```python
from build123d import *

# Parameters (mm, degrees)
BOSS_EXTRUDE1_DEPTH = 5
CUT_EXTRUDE1_DEPTH  = 15
CUT_EXTRUDE4_DEPTH  = 15
SKETCH7_R           = 1
BOSS_EXTRUDE2_DEPTH = 60
SKETCH8_R           = 0.873363885
CUT_EXTRUDE5_DEPTH  = 15
SKETCH9_R           = 0.918957051
CUT_EXTRUDE6_DEPTH  = 15
SKETCH10_R          = 0.859226697
CUT_EXTRUDE7_DEPTH  = 15
SKETCH11_R          = 0.786945752
CUT_EXTRUDE8_DEPTH  = 15


with BuildPart() as part:
    # Sketch1 → Boss-Extrude1 (new body)
    with BuildSketch(Plane(origin=(0, 0, 0), x_dir=(1, 0, 0), z_dir=(0, 1, 0))):
        with BuildLine():
            Line((-35.448928743, 52.732943935), (-27.948927155, 60.232942347))
            ThreePointArc((-27.948927155, 60.232942347), (-7.948927155, 52.732942347), (12.051072845, 60.232942347))
            Line((12.051072845, 60.232942347), (19.551072845, 52.732939171))
            ThreePointArc((19.551072845, 52.732939171), (12.051076647, 32.732945116), (19.551072845, 12.73295106))
            Line((19.551072845, 12.73295106), (12.051060957, 5.232942347))
            ThreePointArc((12.051060957, 5.232942347), (5.043506988, 9.818456658), (-2.948938922, 12.319169055))
            ThreePointArc((-2.948938922, 12.319169055), (-7.948938922, 12.848178709), (-12.948938922, 12.319169055))
            ThreePointArc((-12.948938922, 12.319169055), (-20.941384832, 9.818456658), (-27.9489388, 5.232942347))
            Line((-27.9489388, 5.232942347), (-35.448937212, 12.732943935))
            ThreePointArc((-35.448937212, 12.732943935), (-27.948932978, 32.732942347), (-35.448928743, 52.732943935))
        make_face()
    extrude(amount=BOSS_EXTRUDE1_DEPTH)

    # Sketch3 → Cut-Extrude1 (cut)
    with BuildSketch(Plane(origin=(0, 5, 0), x_dir=(1, 0, 0), z_dir=(0, 1, 0))):
        with BuildLine():
            Line((-27.948927155, 60.232942347), (-35.448928743, 52.732943935))
            ThreePointArc((-35.448928743, 52.732943935), (-27.948932978, 32.732942347), (-35.448937212, 12.732943935))
            Line((-35.448937212, 12.732943935), (-27.9489388, 5.232942347))
            ThreePointArc((-27.9489388, 5.232942347), (-7.948938922, 12.848178709), (12.051060957, 5.232942347))
            Line((12.051060957, 5.232942347), (19.551072845, 12.73295106))
            ThreePointArc((19.551072845, 12.73295106), (12.051076647, 32.732945116), (19.551072845, 52.732939171))
            Line((19.551072845, 52.732939171), (12.051072845, 60.232942347))
            ThreePointArc((12.051072845, 60.232942347), (-7.948927155, 52.732942347), (-27.948927155, 60.232942347))
        make_face()
        with BuildLine():
            Line((-33.493710626, 12.732943935), (-27.9489388, 7.18817211))
            ThreePointArc((-27.9489388, 7.18817211), (-7.948938922, 14.210022681), (12.051060957, 7.18817211))
            Line((12.051060957, 7.18817211), (17.099712422, 12.236821437))
            ThreePointArc((17.099712422, 12.236821437), (10.006359282, 32.484880304), (17.099712422, 52.732939171))
            Line((17.099712422, 52.732939171), (12.051072845, 57.781578748))
            ThreePointArc((12.051072845, 57.781578748), (-7.948927155, 51.108457819), (-27.948927155, 57.781578748))
            Line((-27.948927155, 57.781578748), (-33.493710626, 52.732943935))
            ThreePointArc((-33.493710626, 52.732943935), (-26.205843846, 32.732943935), (-33.493710626, 12.732943935))
        make_face(mode=Mode.SUBTRACT)
    extrude(amount=-CUT_EXTRUDE1_DEPTH, mode=Mode.SUBTRACT)


with BuildPart() as cut_extrude1_kept_piece:
    # of the separate pieces the step leaves, the one the design keeps (cut_extrude1_pieces_kept)
    add(part.part.solids().sort_by_distance((-27.9489388, 0, -7.18817211))[0])

    # Sketch4 → Cut-Extrude4 (cut)
    with BuildSketch(Plane(origin=(0, 5, 0), x_dir=(1, 0, 0), z_dir=(0, 1, 0))):
        with BuildLine():
            Line((-19.583778872, 20.459711597), (-16.194704715, 20.459711597))
            ThreePointArc((-16.194704715, 20.459711597), (-14.85807522, 21.796341092), (-16.194704715, 23.132970587))
            Line((-16.194704715, 23.132970587), (-19.583778872, 23.132970587))
            ThreePointArc((-19.583778872, 23.132970587), (-20.920408367, 21.796341092), (-19.583778872, 20.459711597))
        make_face()
        with BuildLine():
            ThreePointArc((-21.831761669, 21.796341092), (-21.78134565, 17.350791516), (-17.335796074, 17.401207535))
            ThreePointArc((-17.335796074, 17.401207535), (-15.079204869, 17.426799049), (-15.053613355, 15.170207843))
            ThreePointArc((-15.053613355, 15.170207843), (-24.012345341, 15.068608797), (-24.113944388, 24.027340783))
            ThreePointArc((-24.113944388, 24.027340783), (-21.857353183, 24.052932297), (-21.831761669, 21.796341092))
        make_face()
        with BuildLine():
            ThreePointArc((-17.153953535, 47.057082623), (-21.758601657, 47.312085175), (-22.013604209, 42.707437053))
            ThreePointArc((-22.013604209, 42.707437053), (-22.114274365, 40.88960957), (-23.932101848, 40.990279726))
            ThreePointArc((-23.932101848, 40.990279726), (-23.475758984, 49.230582815), (-15.235455895, 48.77423995))
            ThreePointArc((-15.235455895, 48.77423995), (-15.336126051, 46.956412467), (-17.153953535, 47.057082623))
        make_face()
        with BuildLine():
            ThreePointArc((-18.867938752, 44.161713483), (-20.322215182, 42.707437053), (-18.867938752, 41.253160623))
            Line((-18.867938752, 41.253160623), (-17.153953535, 41.253160623))
            ThreePointArc((-17.153953535, 41.253160623), (-15.699677105, 42.707437053), (-17.153953535, 44.161713483))
            Line((-17.153953535, 44.161713483), (-18.867938752, 44.161713483))
        make_face()
        with BuildLine():
            Line((-8.881617516, 44.161713483), (-8.881617516, 19.598774313))
            ThreePointArc((-8.881617516, 19.598774313), (-7.948927155, 18.666083952), (-7.016236793, 19.598774313))
            Line((-7.016236793, 19.598774313), (-7.016236793, 44.161713483))
            ThreePointArc((-7.016236793, 44.161713483), (-7.948927155, 45.094403844), (-8.881617516, 44.161713483))
        make_face()
        with BuildLine():
            Line((-22.013604209, 33.925546285), (5.888104042, 33.925546285))
            ThreePointArc((5.888104042, 33.925546285), (7.080706392, 32.732943935), (5.888104042, 31.540341586))
            Line((5.888104042, 31.540341586), (-22.013604209, 31.540341586))
            ThreePointArc((-22.013604209, 31.540341586), (-23.206206558, 32.732943935), (-22.013604209, 33.925546285))
        make_face()
        with BuildLine():
            ThreePointArc((6.501599793, 42.67386899), (5.971735558, 47.620514921), (1.025089628, 47.090650686))
            ThreePointArc((1.025089628, 47.090650686), (-0.822878242, 46.892704018), (-1.02082491, 48.740671887))
            ThreePointArc((-1.02082491, 48.740671887), (7.621756759, 49.666429458), (8.54751433, 41.023847789))
            ThreePointArc((8.54751433, 41.023847789), (6.699546461, 40.825901121), (6.501599793, 42.67386899))
        make_face()
        with BuildLine():
            ThreePointArc((1.638585378, 41.548852695), (3.515318655, 43.425585972), (1.638585378, 45.302319249))
            Line((1.638585378, 45.302319249), (0.002132359, 45.302319249))
            ThreePointArc((0.002132359, 45.302319249), (-1.874600919, 43.425585972), (0.002132359, 41.548852695))
            Line((0.002132359, 41.548852695), (1.638585378, 41.548852695))
        make_face()
        with BuildLine():
            ThreePointArc((7.510988879, 23.827432924), (5.783954474, 23.723283356), (5.888104042, 21.996248951))
            ThreePointArc((5.888104042, 21.996248951), (6.160819348, 17.474014981), (1.638585378, 17.201299676))
            ThreePointArc((1.638585378, 17.201299676), (-0.088449027, 17.097150108), (0.015700541, 15.370115703))
            ThreePointArc((0.015700541, 15.370115703), (7.992003321, 15.851130144), (7.510988879, 23.827432924))
        make_face()
        with BuildLine():
            ThreePointArc((1.638585378, 18.510682614), (2.726677077, 19.598774313), (1.638585378, 20.686866012))
            Line((1.638585378, 20.686866012), (-0.516238104, 20.686866012))
            ThreePointArc((-0.516238104, 20.686866012), (-1.604329803, 19.598774313), (-0.516238104, 18.510682614))
            Line((-0.516238104, 18.510682614), (1.638585378, 18.510682614))
        make_face()
    extrude(amount=-CUT_EXTRUDE4_DEPTH, mode=Mode.SUBTRACT)

    # Sketch7 → Boss-Extrude2 (add)
    with BuildSketch(Plane(origin=(0, 5, 0), x_dir=(1, 0, 0), z_dir=(0, 1, 0))):
        with Locations(Location((-29.113038054, 52.732942347, 0), (0, 0, 270))):
            Circle(SKETCH7_R)
        with Locations(Location((10.886963534, 52.732942347, 0), (0, 0, 270))):
            Circle(SKETCH7_R)
        with Locations(Location((10.886963534, 12.732942347, 0), (0, 0, 270))):
            Circle(SKETCH7_R)
        with Locations(Location((-29.113046524, 12.732942347, 0), (0, 0, 270))):
            Circle(SKETCH7_R)
    extrude(amount=BOSS_EXTRUDE2_DEPTH)

    # Sketch8 → Cut-Extrude5 (cut)
    with BuildSketch(Plane(origin=(0, 65, 0), x_dir=(1, 0, 0), z_dir=(0, 1, 0))):
        with Locations(Location((-29.113038054, 52.732942347, 0), (0, 0, 270))):
            Circle(SKETCH8_R)
    extrude(amount=-CUT_EXTRUDE5_DEPTH, mode=Mode.SUBTRACT)

    # Sketch9 → Cut-Extrude6 (cut)
    with BuildSketch(Plane(origin=(0, 65, 0), x_dir=(1, 0, 0), z_dir=(0, 1, 0))):
        with Locations(Location((10.886963534, 52.732942347, 0), (0, 0, 270))):
            Circle(SKETCH9_R)
    extrude(amount=-CUT_EXTRUDE6_DEPTH, mode=Mode.SUBTRACT)

    # Sketch10 → Cut-Extrude7 (cut)
    with BuildSketch(Plane(origin=(0, 65, 0), x_dir=(1, 0, 0), z_dir=(0, 1, 0))):
        with Locations(Location((-29.113046524, 12.732942347, 0), (0, 0, 270))):
            Circle(SKETCH10_R)
    extrude(amount=-CUT_EXTRUDE7_DEPTH, mode=Mode.SUBTRACT)

    # Sketch11 → Cut-Extrude8 (cut)
    with BuildSketch(Plane(origin=(0, 65, 0), x_dir=(1, 0, 0), z_dir=(0, 1, 0))):
        with Locations(Location((10.886963534, 12.732942347, 0), (0, 0, 270))):
            Circle(SKETCH11_R)
    extrude(amount=-CUT_EXTRUDE8_DEPTH, mode=Mode.SUBTRACT)


solid = cut_extrude1_kept_piece.part
```
Design review of the part built by this model. Coordinates are the model's own, in mm. A direction names the side the tool comes from. Round coordinates to 2 decimals unless told otherwise and drop trailing zeros. Order: outer loops, then holes, each group sorted by start corner. A loop starts at its lowest first (then second) coordinate and runs counter-clockwise, first axis right, second up. Notation, with made-up numbers: M 43.25,43.5 L 69.25,43.5 A25 ccw 69.25,82.5 Z; hole C 43,-10 d6. An arc over 180 degrees is marked long. Put each result on its own line as item: value.
Q1. Consider section A-A (z = -33). State the section outline as (x, y) points, and give its area (3 significant figures).
Reported:
outline: M -26.21,0 L -23.18,0 L -23.18,5 L -26.21,5 Z; M 7.05,0 L 10.01,0 L 10.01,5 L 7.05,5 Z
area: 30.0 mm²
Q2. Consider section C-C (x = -4). State the section outline as (y, z) points.
Reported:
outline: M 0,-51.34 L 5,-51.34 L 5,-33.93 L 0,-33.93 Z; M 0,-31.54 L 5,-31.54 L 5,-13.97 L 0,-13.97 Z
Q3. Machinability: for faces 1 (the face through (7.08, 2.54, -32.76)), 2 (the face through (-8.25, 2.54, -14.21)), 3 (the face through (-30, 34.58, -12.27)), which of the approach directions +Z, -Z, +X, -X, +Y, -Y give a long, thin tool a straight path to every point of the face, cutting with its end or side? Answer none if there is none.
Reported:
face 1: +Y, -Y
face 2: +Z, +Y, -Y
face 3: +Y
Q4. Draft analysis for pull direction X (two halves, no side actions). For faces 4 (the face through (-23.57, 2.535, -49.144)), 5 (the face through (-30.683, 2.535, -55.293)), state which applies: released by +X, released by -X, zero draft, split by the parting line, or undercut.
Reported:
face 4: undercut
face 5: released by -X
Q5. Consider section D-D (y = 16.5). State the section outline as (x, z) points, and give its area (3 significant figures).
Reported:
outline: C -29.11,-52.73 d2; C -29.11,-12.73 d2; C 10.89,-52.73 d2; C 10.89,-12.73 d2
area: 12.6 mm²
Q6. Consider section B-B (x = 4.5). State the section outline as (y, z) points, and give its area (3 significant figures).
Reported:
outline: M 0,-53.52 L 5,-53.52 L 5,-50.98 L 0,-50.98 Z; M 0,-48.32 L 5,-48.32 L 5,-33.93 L 0,-33.93 Z; M 0,-31.54 L 5,-31.54 L 5,-16.48 L 0,-16.48 Z; M 0,-14 L 5,-14 L 5,-11.69 L 0,-11.69 Z
area: 172 mm²
Q7. Insertion check: pin 1 Ø4 at (x, y) = (-2.5, 1.5) entering from +Z; pin 2 Ø1.8 at (x, y) = (1, 3) entering from -Z; pin 3 Ø2.5 at (x, y) = (-18, 2.5) entering from -Z; pin 4 Ø0.9 at (x, z) = (-29.5, -53) entering from +Y. Each pin has a flat end and moves straight along its axis. Give the tip position at first contact, or say it passes through.
Reported:
pin 1: z = -13.33
pin 2: z = -52.6
pin 3: z = -53.08
pin 4: y = 65
Q8. To check wall thickness, follow line 1 (Y direction, x = -2, z = -24.5); line 2 (Z direction, x = -29, y = 11); line 3 (X direction, y = 21.5, z = -13.5). State the ranges of each line that lie inside material, in increasing order.
Reported:
line 1: 0 to 5
line 2: -53.73 to -51.74, -13.73 to -11.74
line 3: -29.75 to -28.47, 10.25 to 11.53
